from build123d import *

# Parameters (mm, degrees)
BOSS_EXTRUDE1_DEPTH = 46
SKETCH2_R           = 3.625
CUT_EXTRUDE1_DEPTH  = 46
SKETCH3_R           = 1.5
CUT_EXTRUDE2_DEPTH  = 10
CUT_EXTRUDE3_DEPTH  = 10


with BuildPart() as part:
    # Sketch1 → Boss-Extrude1 (new body)
    with BuildSketch(Plane.XY):
        Polygon((0, 0), (30, 0), (30, 3), (3, 3), (3, 38), (0, 38), align=None)
    extrude(amount=BOSS_EXTRUDE1_DEPTH)

    # Sketch2 → Cut-Extrude1 (cut)
    with BuildSketch(Plane(origin=(3, 0, 0), x_dir=(0, 0, -1), z_dir=(1, 0, 0))):
        with Locations((-15, 22)):
            Circle(SKETCH2_R)
        with Locations((-31, 22)):
            Circle(SKETCH2_R)
    extrude(amount=-CUT_EXTRUDE1_DEPTH, mode=Mode.SUBTRACT)

    # Sketch3 → Cut-Extrude2 (cut)
    with BuildSketch(Plane.ZY):
        with Locations((39.5, 31)):
            Circle(SKETCH3_R)
        with Locations((6.5, 31)):
            Circle(SKETCH3_R)
        with Locations((39.5, 13)):
            Circle(SKETCH3_R)
        with Locations((6.5, 13)):
            Circle(SKETCH3_R)
    extrude(amount=-CUT_EXTRUDE2_DEPTH, mode=Mode.SUBTRACT)

    # Sketch4 → Cut-Extrude3 (cut)
    with BuildSketch(Plane(origin=(0, 3, 0), x_dir=(1, 0, 0), z_dir=(0, 1, 0))):
        with BuildLine():
            Line((9.5, -38), (23.5, -38))
            ThreePointArc((23.5, -38), (24.5, -39), (23.5, -40))
            Line((23.5, -40), (9.5, -40))
            ThreePointArc((9.5, -40), (8.5, -39), (9.5, -38))
        make_face()
        with BuildLine():
            Line((9.5, -6), (23.5, -6))
            ThreePointArc((23.5, -6), (24.5, -7), (23.5, -8))
            Line((23.5, -8), (9.5, -8))
            ThreePointArc((9.5, -8), (8.5, -7), (9.5, -6))
        make_face()
    extrude(amount=-CUT_EXTRUDE3_DEPTH, mode=Mode.SUBTRACT)


solid = part.part
Can you work these out from the model? Positions are in its coordinate system, mm. A direction names the side the tool comes from. Round coordinates to 2 decimals unless told otherwise and drop trailing zeros. Loops run counter-clockwise (first coordinate to the right, second up) from the corner with the lowest first, then second, coordinate; pieces in that order, holes last. Notation, with made-up numbers: (53.25, 51.5) - (75.25, 51.5) arc R17 cw to (75.25, 83.5) - close; hole circle Ø5 at (13, 36). An arc over 180 degrees is marked (long way). Use CSV: the item, a comma, the result in double quotes. Start each with the question number.
1) For faces 1 (the cylindrical face through (24.5, 1.5, 39)), 2 (the flat face through (3, 20, 23)), 3 (the cylindrical face through (1.521, 19.794, 33.877)), which set-ups out of +Z, -Z, +X, -X, +Y, -Y let a thin tool reach every point of the face, with its end or its side?
2) We'd pull the mould along X, two halves only. Please class faces 4 (the flat face through (2, 38, 23)), 5 (the flat face through (0, 19, 23)), 6 (the cylindrical face through (8.5, 1.5, 7)): released by +X, released by -X, zero draft, split by the parting line, or undercut.
3) Please list where these lines run through material, in increasing order: probe 1 along Y at (x, z) = (2.4, 6.5); probe 2 along Y at (x, z) = (0.65, 31) (3 decimals); probe 3 along Y at (x, z) = (2.5, 6). Write a range as [from, to].
4) If we section it at D-D on y = 26.5: Write out the boundary of the cut face in (x, z).
5) If we section it at C-C on z = 24: Write out the boundary of the cut face in (x, y).
6) If we section it at A-A on y = 22: Write out the boundary of the cut face in (x, z) (3 decimals).
7) For pin 1 Ø9.5 at (y, z) = (22, 15) entering from +X; pin 2 Ø8.5 at (y, z) = (22, 31) entering from -X; pin 3 Ø8 at (x, z) = (23, 15) entering from +Y, each with a flat end and sliding along its axis, tell me the tip position at first contact or that it passes through.
8) If we section it at B-B on x = 18: Write out the boundary of the cut face in (y, z), plus the area to 3 significant figures.
Geometry results:
1,face 1,"+Y, -Y"
1,face 2,"+Z, -Z, +X, +Y"
1,face 3,"+X, -X"
2,face 4,"zero draft"
2,face 5,"released by -X"
2,face 6,"undercut"
3,probe 1,"y = [0, 11.5], [14.5, 29.5], [32.5, 38]"
3,probe 2,"y = [0, 18.375], [25.625, 38]"
3,probe 3,"y = [0, 11.59], [14.41, 29.59], [32.41, 38]"
4,outline,"(0, 0) - (3, 0) - (3, 46) - (0, 46) - close"
5,outline,"(0, 0) - (30, 0) - (30, 3) - (3, 3) - (3, 38) - (0, 38) - close"
6,outline,"(0, 0) - (3, 0) - (3, 11.375) - (0, 11.375) - close; (0, 18.625) - (3, 18.625) - (3, 27.375) - (0, 27.375) - close; (0, 34.625) - (3, 34.625) - (3, 46) - (0, 46) - close"
7,pin 1,"stops at x = 3"
7,pin 2,"stops at x = 0"
7,pin 3,"stops at y = 3"
8,outline,"(0, 0) - (3, 0) - (3, 6) - (0, 6) - close; (0, 8) - (3, 8) - (3, 38) - (0, 38) - close; (0, 40) - (3, 40) - (3, 46) - (0, 46) - close"
8,area,"126 mm2"
